Here's how the part is built. I have some questions about the finished solid (model axes, mm). Give positions to 0.01 mm unless a question says otherwise; leave off trailing zeros. Write each question's results on one line, items separated by ' | '. Start each with the question number.
Q1. I'm going to push a flat-ended pin straight in: pin 1 (3 mm diameter, centred on x = -101, z = 3, fed in from -Y). Where does the tip first touch, or does it pass through?
Q2. I need wall thicknesses on line 1 along Y through (x, z) = (-1, 9.5). Which ranges of the line are inside material? Lowest first, please. Write a range as [from, to].
Q3. Imagine slicing it at A-A, the plane z = 8. State how many separate pieces and enclosed holes the cut face has, then the cut area to 3 significant figures.
```python
from build123d import *

# Parameters (mm, degrees)
SKETCH002_W                             = 800
SKETCH002_H                             = 200
PAD001_DEPTH                            = 10
SKETCH003_W                             = 15
SKETCH003_H                             = 82
POCKET001_DEPTH                         = 1649.364514
POCKET001_DEPTH_BACK                    = 1659.364514
SKETCH003_LINEARPATTERN002_2_W          = 15
SKETCH003_LINEARPATTERN002_2_H          = 82
POCKET001_LINEARPATTERN002_2_DEPTH      = 1649.364514
POCKET001_LINEARPATTERN002_2_DEPTH_BACK = 1659.364514
SKETCH003_LINEARPATTERN002_3_W          = 15
SKETCH003_LINEARPATTERN002_3_H          = 82
POCKET001_LINEARPATTERN002_3_DEPTH      = 1649.364514
POCKET001_LINEARPATTERN002_3_DEPTH_BACK = 1659.364514
SKETCH003_LINEARPATTERN002_4_W          = 15
SKETCH003_LINEARPATTERN002_4_H          = 82
POCKET001_LINEARPATTERN002_4_DEPTH      = 1649.364514
POCKET001_LINEARPATTERN002_4_DEPTH_BACK = 1659.364514
SKETCH003_LINEARPATTERN002_5_W          = 15
SKETCH003_LINEARPATTERN002_5_H          = 82
POCKET001_LINEARPATTERN002_5_DEPTH      = 1649.364514
POCKET001_LINEARPATTERN002_5_DEPTH_BACK = 1659.364514
SKETCH003_LINEARPATTERN002_6_W          = 15
SKETCH003_LINEARPATTERN002_6_H          = 82
POCKET001_LINEARPATTERN002_6_DEPTH      = 1649.364514
POCKET001_LINEARPATTERN002_6_DEPTH_BACK = 1659.364514
SKETCH003_LINEARPATTERN002_7_W          = 15
SKETCH003_LINEARPATTERN002_7_H          = 82
POCKET001_LINEARPATTERN002_7_DEPTH      = 1649.364514
POCKET001_LINEARPATTERN002_7_DEPTH_BACK = 1659.364514
SKETCH003_LINEARPATTERN002_8_W          = 15
SKETCH003_LINEARPATTERN002_8_H          = 82
POCKET001_LINEARPATTERN002_8_DEPTH      = 1649.364514
POCKET001_LINEARPATTERN002_8_DEPTH_BACK = 1659.364514
LINEARPATTERN003_COUNT                  = 8
LINEARPATTERN003_PITCH                  = 49.95


with BuildPart() as part:
    # Sketch002 → Pad001 (new body)
    with BuildSketch(Plane.XY):
        with Locations((0, 100)):
            Rectangle(SKETCH002_W, SKETCH002_H)
    extrude(amount=PAD001_DEPTH)

    # Sketch003 → Pocket001 (cut, two sides)
    with BuildSketch(Plane(origin=(0, 20, 0), x_dir=(1, 0, 0), z_dir=(0, 0, 1))) as pocket001_sk:
        with Locations((0, 41)):
            Rectangle(SKETCH003_W, SKETCH003_H)
    pocket001 = extrude(amount=-POCKET001_DEPTH, mode=Mode.SUBTRACT) + extrude(pocket001_sk.sketch, amount=POCKET001_DEPTH_BACK, mode=Mode.SUBTRACT)

    # Sketch003 LinearPattern002 2 → Pocket001 LinearPattern002 2 (cut, two sides)
    with BuildSketch(Plane(origin=(49.95, 20, 0), x_dir=(1, 0, 0), z_dir=(0, 0, 1))) as pocket001_linearpattern002_2_sk:
        with Locations((0, 41)):
            Rectangle(SKETCH003_LINEARPATTERN002_2_W, SKETCH003_LINEARPATTERN002_2_H)
    pocket001_linearpattern002_2 = extrude(amount=-POCKET001_LINEARPATTERN002_2_DEPTH, mode=Mode.SUBTRACT) + extrude(pocket001_linearpattern002_2_sk.sketch, amount=POCKET001_LINEARPATTERN002_2_DEPTH_BACK, mode=Mode.SUBTRACT)

    # Sketch003 LinearPattern002 3 → Pocket001 LinearPattern002 3 (cut, two sides)
    with BuildSketch(Plane(origin=(99.9, 20, 0), x_dir=(1, 0, 0), z_dir=(0, 0, 1))) as pocket001_linearpattern002_3_sk:
        with Locations((0, 41)):
            Rectangle(SKETCH003_LINEARPATTERN002_3_W, SKETCH003_LINEARPATTERN002_3_H)
    pocket001_linearpattern002_3 = extrude(amount=-POCKET001_LINEARPATTERN002_3_DEPTH, mode=Mode.SUBTRACT) + extrude(pocket001_linearpattern002_3_sk.sketch, amount=POCKET001_LINEARPATTERN002_3_DEPTH_BACK, mode=Mode.SUBTRACT)

    # Sketch003 LinearPattern002 4 → Pocket001 LinearPattern002 4 (cut, two sides)
    with BuildSketch(Plane(origin=(149.85, 20, 0), x_dir=(1, 0, 0), z_dir=(0, 0, 1))) as pocket001_linearpattern002_4_sk:
        with Locations((0, 41)):
            Rectangle(SKETCH003_LINEARPATTERN002_4_W, SKETCH003_LINEARPATTERN002_4_H)
    pocket001_linearpattern002_4 = extrude(amount=-POCKET001_LINEARPATTERN002_4_DEPTH, mode=Mode.SUBTRACT) + extrude(pocket001_linearpattern002_4_sk.sketch, amount=POCKET001_LINEARPATTERN002_4_DEPTH_BACK, mode=Mode.SUBTRACT)

    # Sketch003 LinearPattern002 5 → Pocket001 LinearPattern002 5 (cut, two sides)
    with BuildSketch(Plane(origin=(199.8, 20, 0), x_dir=(1, 0, 0), z_dir=(0, 0, 1))) as pocket001_linearpattern002_5_sk:
        with Locations((0, 41)):
            Rectangle(SKETCH003_LINEARPATTERN002_5_W, SKETCH003_LINEARPATTERN002_5_H)
    pocket001_linearpattern002_5 = extrude(amount=-POCKET001_LINEARPATTERN002_5_DEPTH, mode=Mode.SUBTRACT) + extrude(pocket001_linearpattern002_5_sk.sketch, amount=POCKET001_LINEARPATTERN002_5_DEPTH_BACK, mode=Mode.SUBTRACT)

    # Sketch003 LinearPattern002 6 → Pocket001 LinearPattern002 6 (cut, two sides)
    with BuildSketch(Plane(origin=(249.75, 20, 0), x_dir=(1, 0, 0), z_dir=(0, 0, 1))) as pocket001_linearpattern002_6_sk:
        with Locations((0, 41)):
            Rectangle(SKETCH003_LINEARPATTERN002_6_W, SKETCH003_LINEARPATTERN002_6_H)
    pocket001_linearpattern002_6 = extrude(amount=-POCKET001_LINEARPATTERN002_6_DEPTH, mode=Mode.SUBTRACT) + extrude(pocket001_linearpattern002_6_sk.sketch, amount=POCKET001_LINEARPATTERN002_6_DEPTH_BACK, mode=Mode.SUBTRACT)

    # Sketch003 LinearPattern002 7 → Pocket001 LinearPattern002 7 (cut, two sides)
    with BuildSketch(Plane(origin=(299.7, 20, 0), x_dir=(1, 0, 0), z_dir=(0, 0, 1))) as pocket001_linearpattern002_7_sk:
        with Locations((0, 41)):
            Rectangle(SKETCH003_LINEARPATTERN002_7_W, SKETCH003_LINEARPATTERN002_7_H)
    pocket001_linearpattern002_7 = extrude(amount=-POCKET001_LINEARPATTERN002_7_DEPTH, mode=Mode.SUBTRACT) + extrude(pocket001_linearpattern002_7_sk.sketch, amount=POCKET001_LINEARPATTERN002_7_DEPTH_BACK, mode=Mode.SUBTRACT)

    # Sketch003 LinearPattern002 8 → Pocket001 LinearPattern002 8 (cut, two sides)
    with BuildSketch(Plane(origin=(349.65, 20, 0), x_dir=(1, 0, 0), z_dir=(0, 0, 1))) as pocket001_linearpattern002_8_sk:
        with Locations((0, 41)):
            Rectangle(SKETCH003_LINEARPATTERN002_8_W, SKETCH003_LINEARPATTERN002_8_H)
    pocket001_linearpattern002_8 = extrude(amount=-POCKET001_LINEARPATTERN002_8_DEPTH, mode=Mode.SUBTRACT) + extrude(pocket001_linearpattern002_8_sk.sketch, amount=POCKET001_LINEARPATTERN002_8_DEPTH_BACK, mode=Mode.SUBTRACT)

    # LinearPattern003: Pocket001, Pocket001 LinearPattern002 2, Pocket001 LinearPattern002 3, Pocket001 LinearPattern002 4, Pocket001 LinearPattern002 5, Pocket001 LinearPattern002 6, Pocket001 LinearPattern002 7, Pocket001 LinearPattern002 8 ×8
    with Locations(*[(-i * LINEARPATTERN003_PITCH, 0, 0) for i in range(1, LINEARPATTERN003_COUNT)]):
        add(pocket001, mode=Mode.SUBTRACT)
        add(pocket001_linearpattern002_2, mode=Mode.SUBTRACT)
        add(pocket001_linearpattern002_3, mode=Mode.SUBTRACT)
        add(pocket001_linearpattern002_4, mode=Mode.SUBTRACT)
        add(pocket001_linearpattern002_5, mode=Mode.SUBTRACT)
        add(pocket001_linearpattern002_6, mode=Mode.SUBTRACT)
        add(pocket001_linearpattern002_7, mode=Mode.SUBTRACT)
        add(pocket001_linearpattern002_8, mode=Mode.SUBTRACT)


solid = part.part
```
Geometry check:
1) pin 1: y = 0
2) line 1: [0, 20], [102, 200]
3) separate pieces: 1 | enclosed holes: 15 | area: 142,000 mm²
